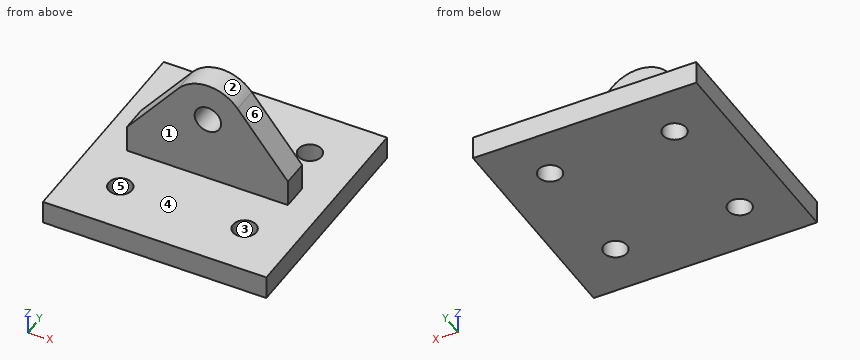
from build123d import *

# Parameters (mm, degrees)
F1_DEPTH = 18.034
F2_W     = 152.4
F2_H     = 152.4
F3_DEPTH = 15.875
F4_D     = 18.034
F5_D     = 15.875


with BuildPart() as f1:
    # F0 (on Front) → F1 (new body)
    with BuildSketch(Plane.XZ):
        with BuildLine():
            Line((0, 18.034), (0, 0))
            Line((0, 0), (109.982, 0))
            Line((109.982, 0), (109.982, 18.034))
            Line((109.982, 18.034), (75.5805723786, 61.1226751156))
            ThreePointArc((75.5805723786, 61.1226751156), (55.4585614287, 70.8657000818), (35.2437223557, 61.316766036))
            Line((35.2437223557, 61.316766036), (0, 18.034))
        make_face()
    extrude(amount=F1_DEPTH)

    # F2 (on Top) → F3 (join)
    with BuildSketch(Plane.XY):
        with Locations((55.3339, -9.017)):
            Rectangle(F2_W, F2_H)
    extrude(amount=-F3_DEPTH)

    # F4 (through all)
    with Locations(Plane(origin=(0, 0, 0), x_dir=(1, 0, 0), z_dir=(0, 1, 0))):
        with Locations((55.3339, -44.958)):
            Hole(F4_D / 2)

    # F5 (through all)
    with Locations(Plane.XY):
        with Locations((97.7519, -50.165), (12.9159, -50.165), (12.9159, 32.131), (97.7519, 32.385)):
            Hole(F5_D / 2)


solid = f1.part
Design review of the part built by this model. Coordinates are the model's own, in mm. Face numbers are marked on the shaded views. A direction names the side the tool comes from. Give positions to 0.01 mm unless a question says otherwise; leave off trailing zeros. Loops run counter-clockwise (first coordinate to the right, second up) from the corner with the lowest first, then second, coordinate; pieces in that order, holes last. Notation, with made-up numbers: (59, 7.5) - (111, 7.5) arc R24 ccw to (111, 23.5) - close; hole circle Ø6 at (62, 27). An arc over 180 degrees is marked (long way). Use CSV: the item, a comma, the result in double quotes. Start each with the question number.
1. Add section D-D (x = 43). State the section outline as (y, z) points (3 decimals), plus the area to 3 significant figures.
2. Add section C-C (y = -3.5). State the section outline as (x, z) points (3 decimals), plus the area to 3 significant figures.
3. Machinability: for the marked faces 1 and 2, which of the approach directions +Z, -Z, +X, -X, +Y, -Y give a long, thin tool a straight path to every point of the face, cutting with its end or side? Answer none if there is none.
4. Wall thickness on L1, parallel to Z at x = 94, y = -59 (3 decimals); L2, parallel to Y at x = 98.5, z = 10.5; L3, parallel to X at y = -7, z = 22.5: over which ranges is each line inside the solid? List them lowest first.
5. Draft analysis for pull direction X (two halves, no side actions). For the marked faces 3, 4, 5 and 6, state which applies: released by +X, released by -X, zero draft, split by the parting line, or undercut.
6. Insertion check: P1, Ø21.5, axis at x = 51, z = 39, coming from the -Y side; P2, Ø3, axis at x = 91.5, y = -4, coming from the +Z side; P3, Ø4, axis at x = 6, y = -46, coming from the +Z side. Each pin has a flat end and moves straight along its axis. Give the tip position at first contact, or say it passes through.
7. Add section A-A (y = -53). State the section outline as (x, z) points (3 decimals).
8. Add section B-B (z = 47). State the section outline as (x, y) points.
Results found:
1,outline,"(-85.217, -15.875) - (67.183, -15.875) - (67.183, 0) - (0, 0) - (0, 67.742) - (-18.034, 67.742) - (-18.034, 0) - (-85.217, 0) - close"
1,area,"3,640 mm²"
2,outline,"(-20.866, -15.875) - (131.534, -15.875) - (131.534, 0) - (109.982, 0) - (109.982, 18.034) - (75.581, 61.123) arc R25.908 ccw to (35.244, 61.317) - (0, 18.034) - (0, 0) - (-20.866, 0) - close; hole circle Ø18.034 at (55.334, 44.958)"
2,area,"7,660 mm²"
3,face 1,"+Z, +X, -X, -Y"
3,face 2,"+Z, +Y, -Y"
4,L1,"z = -15.875 to 0"
4,L2,"y = -18.03 to 0"
4,L3,"x = 3.64 to 106.42"
5,face 3,"undercut"
5,face 4,"zero draft"
5,face 5,"undercut"
5,face 6,"released by +X"
6,P1,"stops at y = -18.03"
6,P2,"stops at z = 43.06"
6,P3,"stops at z = 0"
7,outline,"(-20.866, -15.875) - (5.502, -15.875) - (5.502, 0) - (-20.866, 0) - close; (20.33, -15.875) - (90.338, -15.875) - (90.338, 0) - (20.33, 0) - close; (105.166, -15.875) - (131.534, -15.875) - (131.534, 0) - (105.166, 0) - close"
8,outline,"(23.59, -18.03) - (46.55, -18.03) - (46.55, 0) - (23.59, 0) - close; (64.12, -18.03) - (86.86, -18.03) - (86.86, 0) - (64.12, 0) - close"
